The listing builds one solid part. Answer for the finished solid, in the listing's coordinates (mm). A direction names the side the tool comes from. Round coordinates to 2 decimals unless told otherwise and drop trailing zeros. Write each loop counter-clockwise with the first axis right and the second up, starting at its lowest first coordinate (ties: lowest second). Pieces come first, ordered by that corner, then holes.
Item 1: For a pull along Y with two mould halves and no side action, classify faces 4 (the face through (1.499, 16, 2)), 5 (the face through (51, 12.192, 3)) as +Y half, -Y half, draft (parallel to the pull), parting line (faces both ways), or undercut.
Item 2: Find section B-B on z = 1. Give the number of separate pieces and of enclosed holes in the cut face, then the cut area to 3 significant figures.
Item 3: Find the intervals of material crossed by probe 1 along X at (y, z) = (26.75, 2.5); probe 2 along X at (y, z) = (17, 3.75); probe 3 along Y at (x, z) = (45.5, 1.25) (3 decimals), in increasing order.
Item 4: Find section A-A on x = 66. Give the vertices of the cut face in (y, z) (3 decimals), then the cut area to 3 significant figures.
Item 5: Each of these flat-tipped pins is pushed along its axis until it touches: pin 1 (2.5 mm diameter, centred on x = 93.599, y = 24.003, fed in from +Z); pin 2 (1.6 mm diameter, centred on x = 8.5, y = 15.5, fed in from -Z). Where does it stop, or does it pass through?
Item 6: A tool of negligible diameter and unlimited length cuts with its end or side. For faces 1 (the face through (11.693, 14.354, 7.602)), 2 (the face through (31.75, 16, 3)), 3 (the face through (7.68, 21.56, 1.73)), from which of +Z, -Z, +X, -X, +Y, -Y can it reach the whole face along a straight path? Write none if from no direction.
Item 7: Find section C-C on x = 19. Give the vertices of the cut face in (y, z) (3 decimals).
```python
from build123d import *

# Parameters (mm, degrees)
F0_W      = 101.6
F0_H      = 32.004
F1_DEPTH  = 6.35
F2_R      = 2.372595
F3_DEPTH  = 3.048
F4_R      = 0.508
F5_W      = 13.0048
F5_H      = 29.0068
F5_R      = 2.465374
F5_R_2    = 1.587812
F6_DEPTH  = 3.5052
F7_W      = 101.6
F7_H      = 3.175
F8_DEPTH  = 6.35
F9_W      = 38.1
F9_H      = 7.62
F10_DEPTH = 6.35


with BuildPart() as f1:
    # F0 (on Top) → F1 (new body)
    with BuildSketch(Plane.XY):
        with Locations((50.8, 16.002)):
            Rectangle(F0_W, F0_H)
    extrude(amount=F1_DEPTH)

    # F2 (on face) → F3 (join)
    with BuildSketch(Plane.XY.offset(6.35)):
        with Locations((12.0015, 20.0025)):
            Circle(F2_R)
        with Locations((12.0015, 12.0015)):
            Circle(F2_R)
        with BuildLine():
            ThreePointArc((6.373095, 12.0015), (5.678178, 13.679178), (4.0005, 14.374095))
            ThreePointArc((4.0005, 14.374095), (2.322822, 10.323822), (6.373095, 12.0015))
        make_face()
        with BuildLine():
            ThreePointArc((4.0005, 17.629905), (5.678178, 18.324822), (6.373095, 20.0025))
            ThreePointArc((6.373095, 20.0025), (2.322822, 21.680178), (4.0005, 17.629905))
        make_face()
    extrude(amount=F3_DEPTH)

    # F4
    f4_edges = [f1.edges().sort_by_distance(p)[0] for p in [
        (9.628905, 20.0025, 9.398),
        (4.0005, 22.375095, 9.398),
        (1.627905, 12.0015, 9.398),
        (9.628905, 12.0015, 9.398),
    ]]
    fillet(f4_edges, radius=F4_R)

    # F5 (on face) → F6 (cut)
    with BuildSketch(Plane(origin=(0, 0, 0), x_dir=(1, 0, 0), z_dir=(0, 0, -1))):
        with Locations((8.001, -16.002)):
            Rectangle(F5_W, F5_H)
        with Locations((8.001, -24.003)):
            Circle(F5_R, mode=Mode.SUBTRACT)
        with Locations((8.001, -16.002)):
            Circle(F5_R, mode=Mode.SUBTRACT)
        with Locations((8.001, -8.001)):
            Circle(F5_R, mode=Mode.SUBTRACT)
        with Locations((93.599, -16.002)):
            Rectangle(F5_W, F5_H)
        with Locations((93.599, -24.003)):
            Circle(F5_R, mode=Mode.SUBTRACT)
        with Locations((93.599, -16.002)):
            Circle(F5_R, mode=Mode.SUBTRACT)
        with Locations((93.599, -8.001)):
            Circle(F5_R, mode=Mode.SUBTRACT)
        with Locations((8.001, -8.001)):
            Circle(F5_R_2)
        with Locations((8.001, -16.002)):
            Circle(F5_R_2)
        with Locations((8.001, -24.003)):
            Circle(F5_R_2)
        with Locations((93.599, -8.001)):
            Circle(F5_R_2)
        with Locations((93.599, -16.002)):
            Circle(F5_R_2)
        with Locations((93.599, -24.003)):
            Circle(F5_R_2)
    extrude(amount=-F6_DEPTH, mode=Mode.SUBTRACT)

    # F7 (on face) → F8 (cut, through all)
    with BuildSketch(Plane(origin=(0, 0, 0), x_dir=(1, 0, 0), z_dir=(0, 0, -1))):
        with Locations((50.8, -30.4165)):
            Rectangle(F7_W, F7_H)
        with Locations((50.8, -1.5875)):
            Rectangle(F7_W, F7_H)
    extrude(amount=-F8_DEPTH, mode=Mode.SUBTRACT)

    # F9 (on face) → F10 (cut, through all)
    with BuildSketch(Plane.XY.offset(6.35)):
        with Locations((50.8, 16.002)):
            Rectangle(F9_W, F9_H)
    extrude(amount=-F10_DEPTH, mode=Mode.SUBTRACT)


solid = f1.part
```
Check values:
1. face 4: draft
1. face 5: undercut
2. separate pieces: 9
2. enclosed holes: 7
2. area: 1,720 mm2
3. probe 1: x = 0 to 1.5, 14.5 to 87.1, 100.1 to 101.6
3. probe 2: x = 0 to 31.75, 69.85 to 101.6
3. probe 3: y = 3.175 to 12.192, 19.812 to 28.829
4. outline: (3.175, 0) - (12.192, 0) - (12.192, 6.35) - (3.175, 6.35) - close; (19.812, 0) - (28.829, 0) - (28.829, 6.35) - (19.812, 6.35) - close
4. area: 115 mm2
5. pin 1: stops at z = 6.35
5. pin 2: stops at z = 3.51
6. face 1: +Z
6. face 2: +Z, -Z
6. face 3: -Z
7. outline: (3.175, 0) - (28.829, 0) - (28.829, 6.35) - (3.175, 6.35) - close
